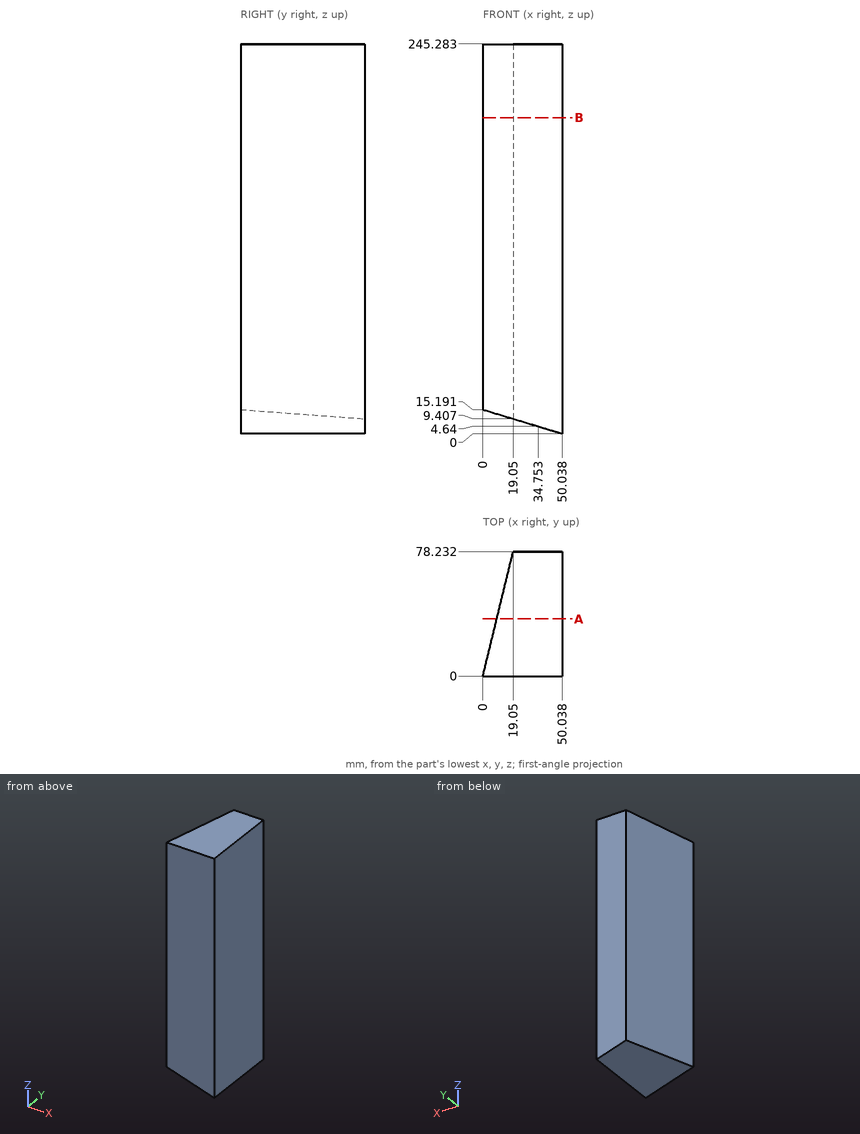
Check sheet for the drawn part. Datum: minimum x, y, z corner. Units: mm. Give positions to 0.01 mm unless a question says otherwise; leave off trailing zeros. Write each loop counter-clockwise with the first axis right and the second up, starting at its lowest first coordinate (ties: lowest second). Pieces come first, ordered by that corner, then holes. Notation, with made-up numbers: (12, -11) -> (21, -11) arc R18 cw to (21, -2) -> close; hole circle Ø9 at (36.5, 9.25). An arc over 180 degrees is marked (long way). Use one line per item in the form item = value. Start each with the question number.
1. Section check A-A (y = 36). Record the cut outline in (x, z).
2. Thickness scan on line 1 along X through (y, z) = (38.5, 101.5) (1 decimal); line 2 along Z through (x, y) = (34, 43); line 3 along Z through (x, y) = (26.5, 68.5) (1 decimal). Record the ranges inside material, lowest first. Write a range as from..to.
3. Go/stop test with flat-tipped pins: P1, Ø2, axis at y = 25.5, z = 164.5, coming from the -X side; P2, Ø1.5, axis at y = 52.5, z = 207.5, coming from the -X side; P3, Ø5, axis at x = 41.5, y = 42.5, coming from the -Z side. Record where each tip stops, or that it passes through.
4. Section check B-B (z = 199). Record the cut outline in (x, y), and give its area (3 significant figures).
Conclusion:
q1.outline = (8.77, 12.53) -> (50.04, 0) -> (50.04, 245.28) -> (8.77, 245.28) -> close
q2.line_1 = 9.4..50
q2.line_2 = 4.87..245.28
q2.line_3 = 7.1..245.3
q3.P1 = 5.97
q3.P2 = 12.6
q3.P3 = 1.83
q4.outline = (0, 0) -> (50.04, 0) -> (50.04, 78.23) -> (19.05, 78.23) -> close
q4.area = 3,170 mm²
